Geometry: final body of the model. Coordinates: model frame, mm. Give positions to 0.01 mm unless a question says otherwise; leave off trailing zeros. Write each loop counter-clockwise with the first axis right and the second up, starting at its lowest first coordinate (ties: lowest second). Pieces come first, ordered by that corner, then holes. Notation, with made-up numbers: M 45.5,23 L 49.5,23 A20 cw 49.5,37 Z; hole C 84,-0.5 d10. An arc over 180 degrees is marked long. One line per question, with ' | ' between items.
Autodesk Fusion 360 part; units mm, degrees
sketch "Sketch1" plane through (0, 0, 0) normal (0, 0, 1) x (1, 0, 0)
  line L0 (0, 0) -> (32.01, 0)
  line L1 (32.01, 0) -> (32.01, 22)
  line L2 (32.01, 22) -> (0, 22)
  line L3 (0, 22) -> (0, 0)
  dimension "d1" = 32.01
  dimension "d2" = 22
extrude "Extrude1" add sketch "Sketch1" along normal blind 1
sketch "Sketch3" plane through (0, 0, 1) normal (0, 0, 1) x (-1, 0, 0)
  line L0 (0, -22) -> (0, 0)
  line L1 (0, 0) -> (-32.01, 0)
  line L2 (-32.01, 0) -> (-32.01, -22)
  line L3 (-32.01, -22) -> (0, -22)
  circle A0 centre (-4.55, -19.5) radius 1
  circle A1 centre (-27.75, -19.5) radius 1
  circle A2 centre (-4.55, -2.49) radius 1
  circle A3 centre (-27.75, -2.49) radius 1
  dimension "d5" = 2
  dimension "d6" = 2.5
  dimension "d7" = 4.55
  dimension "d10" = -23.2
  dimension "d11" = 17.01
extrude "Extrude2" cut sketch "Sketch3" against normal blind 1 contours A0 | A1 | A2 | A3
(1) Cut plane B-B, the plane z = 0.6. Return loops of the section in (x, y), then the cut area to 3 significant figures.
Working result:
outline: M 0,0 L 32.01,0 L 32.01,22 L 0,22 Z; hole C 4.55,2.49 d2; hole C 4.55,19.5 d2; hole C 27.75,2.49 d2; hole C 27.75,19.5 d2 | area: 692 mm^2
(2) Cut plane A-A, the plane x = 4.55. Return loops of the section in (y, z), then the cut area to 3 significant figures.
Working result:
outline: M 0,0 L 1.49,0 L 1.49,1 L 0,1 Z; M 3.49,0 L 18.5,0 L 18.5,1 L 3.49,1 Z; M 20.5,0 L 22,0 L 22,1 L 20.5,1 Z | area: 18.0 mm^2
(3) Material intervals for L1, parallel to X at y = 2.49, z = 0.55; L2, parallel to Y at x = 4.55, z = 0.7, sorted ascending. Write a range as [from, to].
Working result:
L1: x = [0, 3.55], [5.55, 26.75], [28.75, 32.01] | L2: y = [0, 1.49], [3.49, 18.5], [20.5, 22]
(4) Cut plane C-C, the plane y = 19.5. Return loops of the section in (x, z), then the cut area to 3 significant figures.
Working result:
outline: M 0,0 L 3.55,0 L 3.55,1 L 0,1 Z; M 5.55,0 L 26.75,0 L 26.75,1 L 5.55,1 Z; M 28.75,0 L 32.01,0 L 32.01,1 L 28.75,1 Z | area: 28.0 mm^2
(5) Draft query along X for faces 1 (the face through (32.01, 10.8, 0.5)), 2 (the face through (4.767, 20.476, 0.507)), 3 (the face through (0, 11.2, 0.5)), 4 (the face through (16.2, 22, 0.5)). Return one class per face: released by +X, released by -X, zero draft, split by the parting line, or undercut.
Working result:
face 1: released by +X | face 2: undercut | face 3: released by -X | face 4: zero draft
